```python
from build123d import *

# Parameters (mm, degrees)
SKETCH_1_W          = 26
SKETCH_1_H          = 85
EXTRUDE_1_DEPTH     = 2
SKETCH_2_R          = 3
CUT_EXTRUDE_1_DEPTH = 10


with BuildPart() as part:
    # 草图1 → 凸台-拉伸1 (new body)
    with BuildSketch(Plane.XY):
        Rectangle(SKETCH_1_W, SKETCH_1_H)
    extrude_1 = extrude(amount=EXTRUDE_1_DEPTH)

    # 镜向1: 凸台-拉伸1 across plane
    add(extrude_1.mirror(Plane(origin=(14.75, -14.75, 0), x_dir=(0, 0, 1), z_dir=(0.7071067811865488, -0.7071067811865464, 0))))

    # 草图2 → 切除-拉伸1 (cut)
    with BuildSketch(Plane.XY.offset(2)):
        with Locations((0, 22.5)):
            Circle(SKETCH_2_R)
        with Locations((0, 2.5)):
            Circle(SKETCH_2_R)
    cut_extrude_1 = extrude(amount=-CUT_EXTRUDE_1_DEPTH, mode=Mode.SUBTRACT)

    # 镜向2: 切除-拉伸1 across plane
    add(cut_extrude_1.mirror(Plane(origin=(14.75, -14.75, 0), x_dir=(0, 0, 1), z_dir=(0.7071067811865479, -0.7071067811865471, 0))), mode=Mode.SUBTRACT)


solid = part.part
```
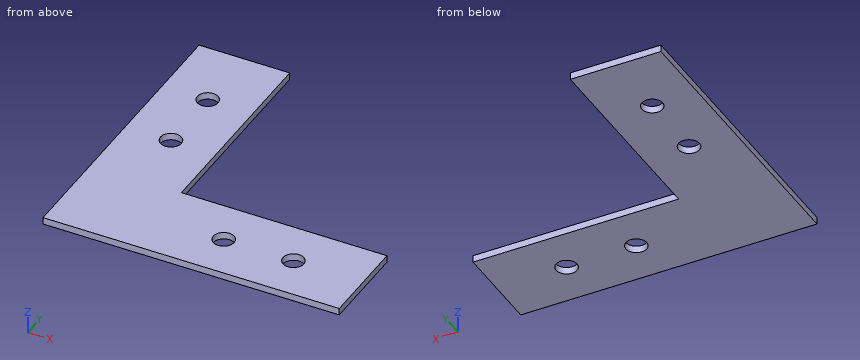
Part model, mm, in its own coordinate system. Coordinates: 2 decimals unless noted, no trailing zeros. Order: outer loops, then holes, each group sorted by start corner. A loop starts at its lowest first (then second) coordinate and runs counter-clockwise, first axis right, second up. Notation, with made-up numbers: (-21, 84.5) - (27, 84.5) arc R17 cw to (27, 110.5) - close; hole circle Ø2 at (52.25, -29.75). An arc over 180 degrees is marked (long way). Return JSON: item names as keys, results as strings. Group by question number.
Item 1: Cut at A-A (y = 2.5). List the corners of the cut face in (x, z), plus the area to 3 significant figures.
Item 2: Pin check, flat tips, straight feed: pin 1 (0.6 mm diameter, centred on x = 49, z = 0.5, fed in from +Y); pin 2 (5 mm diameter, centred on x = 0, y = 2.5, fed in from -Z). Stop position of each tip, or through.
Item 3: Cut at D-D (x = 0). List the corners of the cut face in (y, z), plus the area to 3 significant figures.
Item 4: Cut at C-C (x = 32). List the corners of the cut face in (y, z).
Item 5: Drill centre lines: probe 1 along X at (y, z) = (-29.5, 0.9); probe 2 along Y at (x, z) = (0, 1.25); probe 3 along Y at (x, z) = (22.5, 0.2). Where is each one in solid material? Low to high. Write a range as from..to.
Item 6: Cut at B-B (z = 1). List the corners of the cut face in (x, y), plus the area to 3 significant figures.
Check values:
{
 "1": {"outline": "(-13, 0) - (-3, 0) - (-3, 2) - (-13, 2) - close; (3, 0) - (13, 0) - (13, 2) - (3, 2) - close", "area": "40.0 mm2"},
 "2": {"pin 1": "stops at y = -16.5", "pin 2": "passes through"},
 "3": {"outline": "(-42.5, 0) - (-0.5, 0) - (-0.5, 2) - (-42.5, 2) - close; (5.5, 0) - (19.5, 0) - (19.5, 2) - (5.5, 2) - close; (25.5, 0) - (42.5, 0) - (42.5, 2) - (25.5, 2) - close", "area": "146 mm2"},
 "4": {"outline": "(-42.5, 0) - (-32.5, 0) - (-32.5, 2) - (-42.5, 2) - close; (-26.5, 0) - (-16.5, 0) - (-16.5, 2) - (-26.5, 2) - close"},
 "5": {"probe 1": "x = -13..29, 35..49, 55..72", "probe 2": "y = -42.5..-0.5, 5.5..19.5, 25.5..42.5", "probe 3": "y = -42.5..-16.5"},
 "6": {"outline": "(-13, -42.5) - (72, -42.5) - (72, -16.5) - (13, -16.5) - (13, 42.5) - (-13, 42.5) - close; hole circle Ø6 at (0, 2.5); hole circle Ø6 at (0, 22.5); hole circle Ø6 at (32, -29.5); hole circle Ø6 at (52, -29.5)", "area": "3,630 mm2"}
}
